Autodesk Inventor part; units mm, degrees
ref_plane "YZ Plane" through (0, 0, 0) normal (1, 0, 0) x (0, 1, 0)
ref_plane "XZ Plane" through (0, 0, 0) normal (0, 1, 0) x (-1, 0, 0)
ref_plane "XY Plane" through (0, 0, 0) normal (0, 0, 1) x (1, 0, 0)
sketch "Sketch1" plane through (0, 0, 0) normal (0, 0, 1) x (1, 0, 0)
  circle A0 centre (0, 0) radius 37
  dimension "d0" = 74
extrude "Extrusion1" add sketch "Sketch1" along normal blind 22
sketch "Sketch2" plane through (0, 0, 22) normal (0, 0, 1) x (1, 0, 0)
  circle A0 centre (0, 0) radius 22.5
  dimension "d19" = 45
extrude "Extrusion2" add sketch "Sketch2" along normal blind 7
sketch "Sketch7" plane through (0, 0, 22) normal (0, 0, 1) x (1, 0, 0)
  circle A0 centre (0, 0) radius 22.5
  circle A1 centre (0, 0) radius 24.5
  circle A2 centre (0, 0) radius 37
  circle A3 centre (0, 0) radius 33
  dimension "d12" = 2
  dimension "d13" = 4
extrude "Extrusion5" cut sketch "Sketch7" against normal blind 2 contours A3
sketch "Sketch8" plane through (0, 0, 0) normal (0, 0, -1) x (-1, 0, 0)
  circle A0 centre (0, 0) radius 34
  circle A1 centre (0, 0) radius 37
  dimension "d16" = 3
extrude "Extrusion6" cut sketch "Sketch8" against normal blind 16 contours A0
sketch "Sketch9" plane through (0, 0, 29) normal (0, 0, 1) x (1, 0, 0)
  circle A0 centre (0, 0) radius 7.5
  dimension "d20" = 15
extrude "Extrusion7" cut sketch "Sketch9" against normal blind 29
sketch "Sketch10" plane through (0, 0, 29) normal (0, 0, 1) x (1, 0, 0)
  circle A0 centre (0, 0) radius 17.25
  circle A1 centre (0, 17.25) radius 1.65
  circle A2 centre (-14.938938, 8.625) radius 1.65
  circle A3 centre (-14.938938, -8.625) radius 1.65
  circle A4 centre (0, -17.25) radius 1.65
  circle A5 centre (14.938938, -8.625) radius 1.65
  circle A6 centre (14.938938, 8.625) radius 1.65
  dimension "d23" = 34.5
  dimension "d24" = 3.3
  dimension "d27" = 360
extrude "Extrusion8" cut sketch "Sketch10" against normal through all contours A6 A0 | A0 A6 | A5 A0 | A0 A5 | A1 A0 | A0 A1 | A4 A0 | A0 A4 | A2 A0 | A0 A2 | A3 A0 | A0 A3
sketch "Sketch11" plane through (0, 0, 0) normal (0, 0, -1) x (-1, 0, 0)
  circle A0 centre (0, 0) radius 34
  circle A1 centre (0, 0) radius 37
extrude "Extrusion9" cut sketch "Sketch11" against normal blind 6
chamfer "Chamfer1" distance 4 angle 45 1 edges at (34, 0, 16)
sketch "Sketch12" plane through (0, 0, 22) normal (0, 0, 1) x (1, 0, 0)
  circle A0 centre (0, 0) radius 37
  circle A1 centre (0, 0) radius 33
  circle A2 centre (0, 0) radius 7.5
  circle A3 centre (0, 0) radius 37.75
  dimension "d36" = 0.75
extrude "Extrusion10" add sketch "Sketch12" along normal blind 1 contours A0 | A2 | A3
chamfer "Chamfer3" distance 2 angle 45 2 edges at (-33, 0, 20) (-24.5, 0, 20)
sketch "Sketch14" plane through (0, 0, 6) normal (0, 0, -1) x (-1, 0, 0)
  circle A0 centre (0, 0) radius 37
  circle A1 centre (0, 0) radius 34
  circle A2 centre (0, 0) radius 36.75
  dimension "d47" = 0.25
sketch "Sketch14 outline for Extrusion12" plane through (0, 0, 6) normal (0, 0, -1) x (-1, 0, 0)
  circle A0 centre (0, 0) radius 37
  circle A1 centre (0, 0) radius 36.75
extrude "Extrusion12" cut sketch "Sketch14 outline for Extrusion12" against normal blind 12
sketch "Sketch15" plane through (0, 0, 18) normal (0, 0, -1) x (-1, 0, 0)
  circle A0 centre (0, 0) radius 37
  circle A1 centre (0, 0) radius 36.75
  circle A2 centre (0, 0) radius 36.99
  dimension "d50" = 0.01
sketch "Sketch15 outline for Extrusion13" plane through (0, 0, 18) normal (0, 0, -1) x (-1, 0, 0)
  circle A0 centre (0, 0) radius 37
  circle A1 centre (0, 0) radius 36.99
extrude "Extrusion13" cut sketch "Sketch15 outline for Extrusion13" against normal up to surface (4 mm away)
sketch "Sketch16" plane through (0, 0, 6) normal (0, 0, -1) x (-1, 0, 0)
  circle A0 centre (0, 0) radius 36.75
  circle A1 centre (0, 0) radius 34
extrude "Extrusion14" cut sketch "Sketch16" against normal blind 0.1
sketch "Sketch17" plane through (0, 0, 29) normal (0, 0, 1) x (1, 0, 0)
  circle A0 centre (0, 0) radius 7.5
extrude "Extrusion15" cut sketch "Sketch17" against normal through all
properties part number "rotor_hub"
Read the model definition and answer for the solid it produces. Units are mm, in the model's axes. A direction names the side the tool comes from. Round coordinates to 2 decimals unless told otherwise and drop trailing zeros. Write each loop counter-clockwise with the first axis right and the second up, starting at its lowest first coordinate (ties: lowest second). Pieces come first, ordered by that corner, then holes.
Q1. The mould has two halves that part along Y. Classify faces 4 (the face through (6.56, -29.53, 15.75)), 5 (the face through (10, 0, 29)), 6 (the face through (8.02, -36.11, 19.97)): released by +Y, released by -Y, zero draft, split by the parting line, or undercut.
Values:
face 4: undercut
face 5: zero draft
face 6: split by the parting line
Q2. Find section A-A on z = 24. Determine the outline of the cut face in (x, y) (3 decimals).
Values:
outline: circle Ø45 at (0, 0); hole circle Ø3.3 at (-14.939, -8.625); hole circle Ø3.3 at (-14.939, 8.625); hole circle Ø15 at (0, 0); hole circle Ø3.3 at (0, -17.25); hole circle Ø3.3 at (0, 17.25); hole circle Ø3.3 at (14.939, -8.625); hole circle Ø3.3 at (14.939, 8.625)
Q3. Straight lines are drawn through the part: line 1 (Y direction, x = 0, z = 20.5); line 2 (Y direction, x = 0, z = 9.75); line 3 (Y direction, x = -1, z = 17). For each, find the intervals that lie inside material, in ascending order.
Values:
line 1: y = -36.99 to -31.5, -26 to -18.9, -15.6 to -7.5, 7.5 to 15.6, 18.9 to 26, 31.5 to 36.99
line 2: y = -36.75 to -34, 34 to 36.75
line 3: y = -36.74 to -18.56, -15.94 to -7.43, 7.43 to 15.94, 18.56 to 36.74
Q4. A tool of negligible diameter and unlimited length cuts with its end or side. For faces 1 (the face through (25, -28, 22)), 2 (the face through (30.5, 12.6, 22.5)), 3 (the face through (-7.493, 0.33, 22.591)), from which of +Z, -Z, +X, -X, +Y, -Y can it reach the whole face along a straight path? Write none if from no direction.
Values:
face 1: -Z
face 2: +Z
face 3: +Z, -Z
Q5. Flat-ended cylindrical pins translate along their axes: P1, Ø5, axis at x = -1, z = 8.5, coming from the +Y side; P2, Ø1, axis at x = 14, z = 12, coming from the +Y side; P3, Ø19.5, axis at x = 0, y = 0, coming from the -Z side. Find the tip coordinate at first contact, or state that the pin passes through.
Values:
P1: stops at y = 36.75
P2: stops at y = 34.18
P3: stops at z = 16
